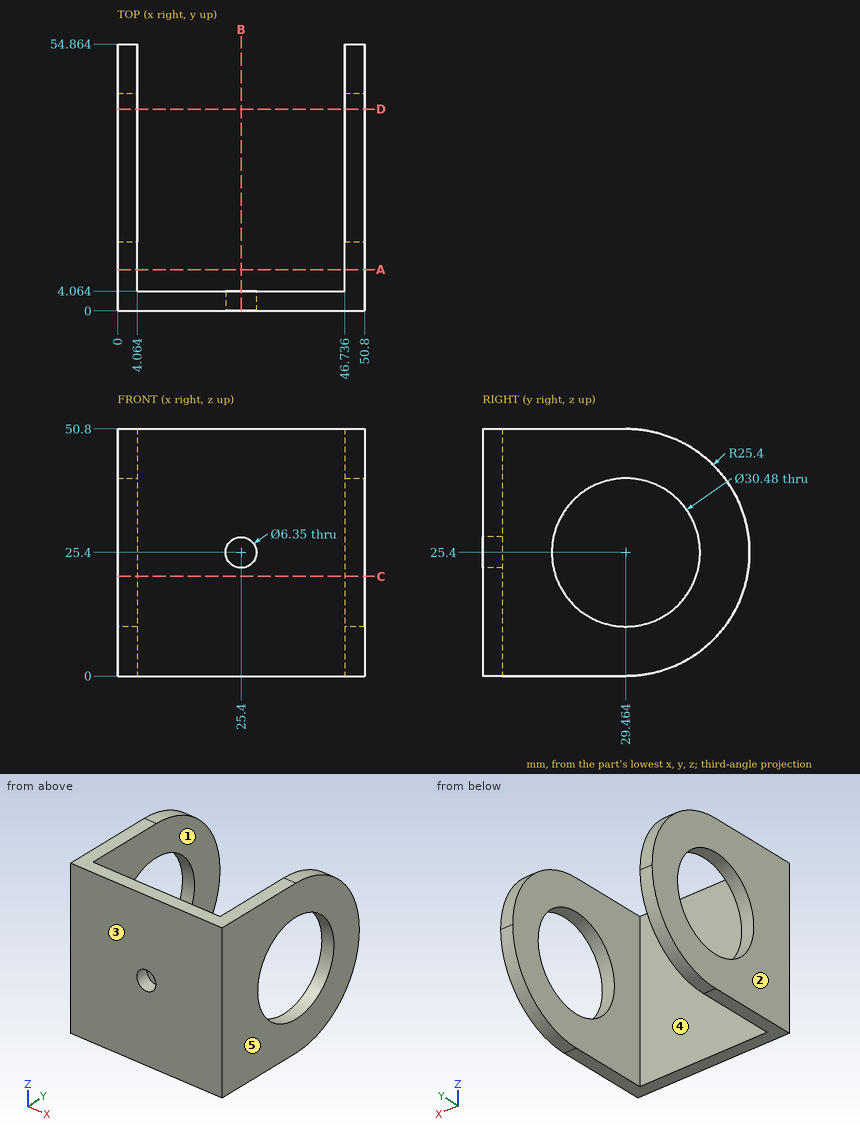
The figure shows three views and two pictorial views of one solid part (mm, origin at its lowest corner). Answer the questions. A direction names the side the tool comes from. Give positions to 0.01 mm unless a question says otherwise; leave off trailing zeros. Order: outer loops, then holes, each group sorted by start corner. A loop starts at its lowest first (then second) coordinate and runs counter-clockwise, first axis right, second up. Notation, with made-up numbers: M -14.75,9 L -2.75,9 A8 ccw -2.75,20 Z; hole C 36.25,-14 d7. An arc over 180 degrees is marked long. Return JSON: item names as keys, results as strings.
1) A tool of negligible diameter and unlimited length cuts with its end or side. For the marked faces 4 and 5, from which of +Z, -Z, +X, -X, +Y, -Y can it reach the whole face along a straight path? Write none if from no direction.
Resolved:
{"face 4": "+Z, -Z, +Y", "face 5": "+Z, -Z, +X, +Y, -Y"}
2) Section D-D, the plane y = 41.5 is taken. Write down the section's boundary in (x, z).
Resolved:
{"outline": "M 0,3.03 L 4.06,3.03 L 4.06,16.05 L 0,16.05 Z; M 0,34.75 L 4.06,34.75 L 4.06,47.77 L 0,47.77 Z; M 46.74,3.03 L 50.8,3.03 L 50.8,16.05 L 46.74,16.05 Z; M 46.74,34.75 L 50.8,34.75 L 50.8,47.77 L 46.74,47.77 Z"}
3) For a pull along X with two mould halves and no side action, classify the marked faces 1, 2 and 3 as +X half, -X half, draft (parallel to the pull), parting line (faces both ways), or undercut.
Resolved:
{"face 1": "undercut", "face 2": "-X half", "face 3": "draft"}
4) Section B-B, the plane x = 25.4 is taken. Write down the section's boundary in (y, z) (3 decimals).
Resolved:
{"outline": "M 0,0 L 4.064,0 L 4.064,22.225 L 0,22.225 Z; M 0,28.575 L 4.064,28.575 L 4.064,50.8 L 0,50.8 Z"}
5) Section A-A, the plane y = 8.5 is taken. Write down the section's boundary in (x, z), plus the area to 3 significant figures.
Resolved:
{"outline": "M 0,0 L 4.06,0 L 4.06,50.8 L 0,50.8 Z; M 46.74,0 L 50.8,0 L 50.8,50.8 L 46.74,50.8 Z", "area": "413 mm^2"}
6) Section C-C, the plane z = 20.5 is taken. Write down the section's boundary in (x, y), plus the area to 3 significant figures.
Resolved:
{"outline": "M 0,0 L 50.8,0 L 50.8,15.03 L 46.74,15.03 L 46.74,4.06 L 4.06,4.06 L 4.06,15.03 L 0,15.03 Z; M 0,43.89 L 4.06,43.89 L 4.06,54.39 L 0,54.39 Z; M 46.74,43.89 L 50.8,43.89 L 50.8,54.39 L 46.74,54.39 Z", "area": "381 mm^2"}
7) Straight lines are drawn through the part: line 1 along X through (y, z) = (5, 14); line 2 along Y through (x, z) = (2.3, 25.4); line 3 along Y through (x, z) = (19, 3). For each, find the intervals that lie inside material, in ascending order. Write a range as [from, to].
Resolved:
{"line 1": "[0, 4.06], [46.74, 50.8]", "line 2": "[0, 14.22], [44.7, 54.86]", "line 3": "[0, 4.06]"}
8) Each of these flat-tipped pins is pushed along its axis until it touches: pin 1 (2 mm diameter, centred on x = 26.5, z = 9, fed in from +Y); pin 2 (24.5 mm diameter, centred on y = 29.464, z = 25.4, fed in from -X). Where does it stop, or does it pass through?
Resolved:
{"pin 1": "y = 4.06", "pin 2": "through"}
